Answer from the drawing. Dimensions are ordinates in mm from the lowest x, y and z of the part. A direction names the side the tool comes from. Round coordinates to 2 decimals unless told otherwise and drop trailing zeros. Loops run counter-clockwise (first coordinate to the right, second up) from the corner with the lowest first, then second, coordinate; pieces in that order, holes last. Notation, with made-up numbers: (55.5, 83.5) -> (75.5, 83.5) arc R14 ccw to (75.5, 108.5) -> close; hole circle Ø7 at (24, 83). An arc over 180 degrees is marked (long way). One line per question, with ' | ' between items.
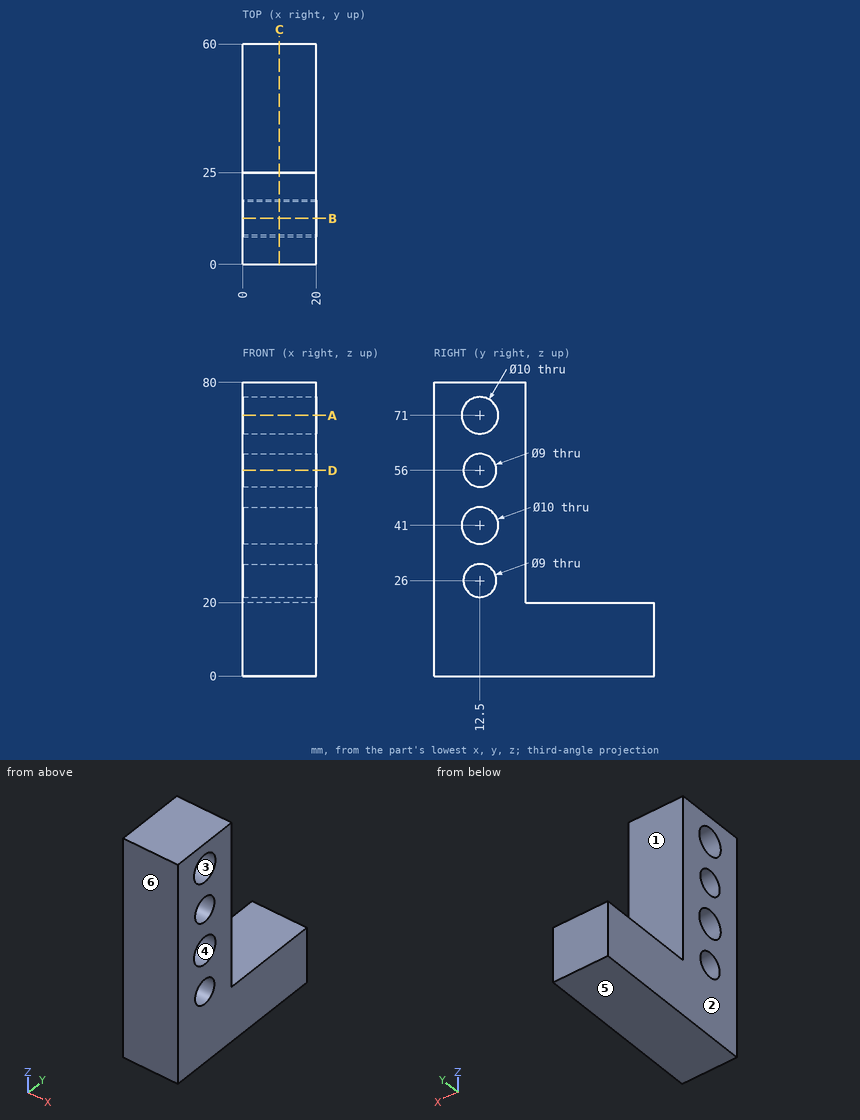
Q1. Given pin 1 Ø4 at (x, z) = (8, 24) entering from -Y; pin 2 Ø8 at (y, z) = (12.5, 71) entering from -X; pin 3 Ø1 at (x, z) = (7, 27.5) entering from +Y, each flat-ended and moving along its own axis, determine where each tip first touches the part or whether it passes through.
Numbers:
pin 1: y = 0 | pin 2: through | pin 3: y = 25
Q2. A cutting plane is placed at C-C on x = 10. Give the vertices of the cut face in (y, z).
Numbers:
outline: (0, 0) -> (60, 0) -> (60, 20) -> (25, 20) -> (25, 80) -> (0, 80) -> close; hole circle Ø10 at (12.5, 41); hole circle Ø10 at (12.5, 71); hole circle Ø9 at (12.5, 26); hole circle Ø9 at (12.5, 56)
Q3. A cutting plane is placed at A-A on z = 71. Give the vertices of the cut face in (x, y).
Numbers:
outline: (0, 0) -> (20, 0) -> (20, 7.5) -> (0, 7.5) -> close; (0, 17.5) -> (20, 17.5) -> (20, 25) -> (0, 25) -> close
Q4. For the marked faces 1 and 2, determine the directions among +Z, -Z, +X, -X, +Y, -Y from which every point of the face is accessible in a straight line to the end or side of a thin tool.
Numbers:
face 1: +Z, +X, -X, +Y | face 2: +Z, -Z, -X, +Y, -Y
Q5. Find the intervals of material crossed by line 1 (Z direction, x = 11.5, y = 12.5); line 2 (Z direction, x = 14.25, y = 54); line 3 (Y direction, x = 9.5, z = 57), in increasing order. Write a range as from..to.
Numbers:
line 1: 0..21.5, 30.5..36, 46..51.5, 60.5..66, 76..80 | line 2: 0..20 | line 3: 0..8.11, 16.89..25
Q6. A cutting plane is placed at D-D on z = 56. Give the vertices of the cut face in (x, y), plus the area to 3 significant figures.
Numbers:
outline: (0, 0) -> (20, 0) -> (20, 8) -> (0, 8) -> close; (0, 17) -> (20, 17) -> (20, 25) -> (0, 25) -> close | area: 320 mm^2
Q7. For a pull along Z with two mould halves and no side action, classify the marked faces 3, 4, 5 and 6 as pulls with the +Z half, pulls with the -Z half, needs draft (parallel to the pull), parting line crosses it, or undercut.
Numbers:
face 3: undercut | face 4: undercut | face 5: pulls with the -Z half | face 6: needs draft
Q8. A cutting plane is placed at B-B on y = 12.5. Give the vertices of the cut face in (x, z), plus the area to 3 significant figures.
Numbers:
outline: (0, 0) -> (20, 0) -> (20, 21.5) -> (0, 21.5) -> close; (0, 30.5) -> (20, 30.5) -> (20, 36) -> (0, 36) -> close; (0, 46) -> (20, 46) -> (20, 51.5) -> (0, 51.5) -> close; (0, 60.5) -> (20, 60.5) -> (20, 66) -> (0, 66) -> close; (0, 76) -> (20, 76) -> (20, 80) -> (0, 80) -> close | area: 840 mm^2
